```python
from build123d import *

# Parameters (mm, degrees)
SZKIC1_R                        = 100
DODANIE_WYCI_GNI_CIE2_DEPTH     = 5
SZKIC2_R                        = 100
SZKIC2_R_2                      = 75
DODANIE_WYCI_GNI_CIE3_DEPTH     = 20
ZAOKR_GLENIE1_R                 = 5
SZKIC4_R                        = 10
WYTNIJ_WYCI_GNI_CIE2_DEPTH      = 5
WYTNIJ_WYCI_GNI_CIE3_DEPTH      = 145.568323017
WYTNIJ_WYCI_GNI_CIE3_DEPTH_BACK = 145.568323017
SZKIC3_R                        = 4.25
SZKIC5_W                        = 6
SZKIC5_H                        = 6
SZKIC6_R                        = 0.6
WYTNIJ_WYCI_GNI_CIE4_DEPTH      = 3


with BuildPart() as part:
    # Szkic1 → Dodanie-wyciągnięcie2 (new, symmetric)
    with BuildSketch(Plane.XY):
        Circle(SZKIC1_R)
    extrude(amount=DODANIE_WYCI_GNI_CIE2_DEPTH, both=True)

    # Szkic2 → Dodanie-wyciągnięcie3 (add)
    with BuildSketch(Plane(origin=(0, 0, -5), x_dir=(-1, 0, 0), z_dir=(0, 0, -1))):
        Circle(SZKIC2_R)
        Circle(SZKIC2_R_2, mode=Mode.SUBTRACT)
    extrude(amount=DODANIE_WYCI_GNI_CIE3_DEPTH)

    # Zaokrąglenie1
    zaokr_glenie1_edges = [part.edges().sort_by_distance(p)[0] for p in [
        (-100, 0, 5),
    ]]
    fillet(zaokr_glenie1_edges, radius=ZAOKR_GLENIE1_R)

    # Szkic4 → Wytnij-wyciągnięcie2 (cut)
    with BuildSketch(Plane.XY.offset(5)):
        Circle(SZKIC4_R)
    extrude(amount=-WYTNIJ_WYCI_GNI_CIE2_DEPTH, mode=Mode.SUBTRACT)

    # Szkic3 → Wytnij-wyciągnięcie3 (cut, two sides: drawn at the far end of the back side and taken through both)
    with BuildSketch(Plane.XY.offset(5).offset(-WYTNIJ_WYCI_GNI_CIE3_DEPTH_BACK)):
        with Locations((87.5, 0)):
            Circle(SZKIC3_R)
        with Locations((0, 87.5)):
            Circle(SZKIC3_R)
        with Locations((0, -87.5)):
            Circle(SZKIC3_R)
        with Locations((-87.5, 0)):
            Circle(SZKIC3_R)
    extrude(amount=WYTNIJ_WYCI_GNI_CIE3_DEPTH + WYTNIJ_WYCI_GNI_CIE3_DEPTH_BACK, mode=Mode.SUBTRACT)

    # Szkic5 → Wycięcie-obrót1 (revolve, cut)
    with BuildSketch(Plane(origin=(0, 0, 0), x_dir=(1, 0, 0), z_dir=(0, 1, 0)), mode=Mode.PRIVATE) as wyci_cie_obr_t1_sk:
        with Locations((-78, 13)):
            Rectangle(SZKIC5_W, SZKIC5_H)
    revolve(wyci_cie_obr_t1_sk.sketch.rotate(Axis((0, 0, 17.369843618), (0, 0, -1)), 180), axis=Axis((0, 0, 17.369843618), (0, 0, -1)), mode=Mode.SUBTRACT)

    # Szkic6 → Wytnij-wyciągnięcie4 (cut)
    with BuildSketch(Plane(origin=(0, 0, -5), x_dir=(-1, 0, 0), z_dir=(0, 0, -1))):
        with Locations((0, -64)):
            Circle(SZKIC6_R)
        with Locations((-64, 0)):
            Circle(SZKIC6_R)
        with Locations((0, 64)):
            Circle(SZKIC6_R)
        with Locations((64, 0)):
            Circle(SZKIC6_R)
    extrude(amount=-WYTNIJ_WYCI_GNI_CIE4_DEPTH, mode=Mode.SUBTRACT)


solid = part.part
```
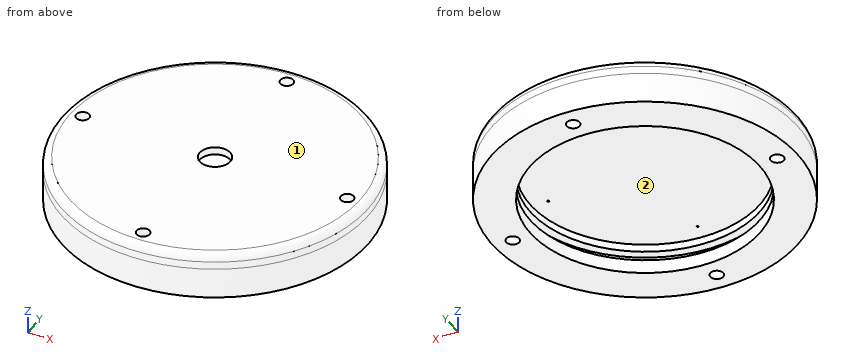
Verification items for the finished model (mm, model axes). Face numbers are marked on the shaded views. Give positions to 0.01 mm unless a question says otherwise; leave off trailing zeros. Order: outer loops, then holes, each group sorted by start corner. A loop starts at its lowest first (then second) coordinate and runs counter-clockwise, first axis right, second up. Notation, with made-up numbers: (56, 27) -> (60, 27) arc R26 cw to (60, 64) -> close; hole circle Ø4 at (43.5, 48.25). An arc over 180 degrees is marked (long way). One line per item, written item: value.
(1) Gauge pin test, flat ends, axial feed: pin 1 (8 mm diameter, centred on y = 49.5, z = -16.5, fed in from -X); pin 2 (0.6 mm diameter, centred on x = 0, y = -64, fed in from -Z); pin 3 (1 mm diameter, centred on y = -68, z = -14, fed in from -X). Record the tip position at first contact, or that the pin passes through.
Final values:
pin 1: x = -89.05
pin 2: z = -2
pin 3: x = -73.78
(2) Sectioned sample at A-A on z = -20.25. Record the cut outline in (x, y).
Final values:
outline: circle Ø200 at (0, 0); hole circle Ø8.5 at (-87.5, 0); hole circle Ø150 at (0, 0); hole circle Ø8.5 at (0, -87.5); hole circle Ø8.5 at (0, 87.5); hole circle Ø8.5 at (87.5, 0)
(3) Scan lines: line 1 along X through (y, z) = (0, -17.75); line 2 along Y through (x, z) = (0, -3.65). Record each from-to range of solid material in increasing order. Write a range as [from, to].
Final values:
line 1: [-100, -91.75], [-83.25, -75], [75, 83.25], [91.75, 100]
line 2: [-100, -91.75], [-83.25, -64.6], [-63.4, 63.4], [64.6, 83.25], [91.75, 100]
(4) Draft check along Y on the marked faces 1 and 2. Enter one of: pulls with the +Y half, pulls with the -Y half, needs draft (parallel to the pull), parting line crosses it, or undercut.
Final values:
face 1: needs draft
face 2: undercut
